Autodesk Inventor part; units mm, degrees
ref_plane "YZ Plane" through (0, 0, 0) normal (1, 0, 0) x (0, 1, 0)
ref_plane "XZ Plane" through (0, 0, 0) normal (0, 1, 0) x (-1, 0, 0)
ref_plane "XY Plane" through (0, 0, 0) normal (0, 0, 1) x (1, 0, 0)
sketch "草圖1" plane through (0, 0, 0) normal (0, 1, 0) x (-1, 0, 0)
  line L0 (0, 0) -> (20, 0)
  line L1 (20, 0) -> (20, 16)
  line L2 (20, 16) -> (0, 16)
  line L3 (0, 16) -> (0, 0)
  dimension "d0" = 20
  dimension "d1" = 16
extrude "擠出1" add sketch "草圖1" along normal blind 11.5
sketch "草圖2" plane through (-20, 0, 16) normal (0, 0, 1) x (1, 0, 0)
  line L0 (0, 0) -> (20, 0)
  line L1 (20, 0) -> (20, 11.5)
  point P0 (16.5, 4.8)
  dimension "d4" = 3.5
  dimension "d5" = 4.8
hole "孔1" at (-3.5, 4.8, 16) direction (0, 0, -1) diameter 2.459 depth 3.5 tip angle 118
sketch "草圖3" plane through (-20, 0, 16) normal (0, 0, 1) x (1, 0, 0)
  line L0 (0, 0) -> (20, 0)
  line L1 (20, 0) -> (20, 11.5)
  point P0 (18, 2)
  dimension "d13" = 2
  dimension "d14" = 2
hole "孔2" at (-2, 2, 16) direction (0, 0, -1) diameter 1.5 depth 4.5 tip angle 118
chamfer "倒角1" distance 0.5 angle 45 12 edges at (-10, 0, 16) (0, 5.75, 16) (0, 0, 8) (-20, 0, 8) (-20, 5.75, 16) (0, 5.75, 0) (-10, 0, 0) (0, 11.5, 8) (-10, 11.5, 16) (-20, 11.5, 8) (-20, 5.75, 0) (-10, 11.5, 0)
sketch "草圖4" plane through (-19.5, 0.5, 16) normal (0, 0, 1) x (1, 0, 0)
  circle A0 centre (8, 3.5) radius 3
  line L0 (0, -0.5) -> (19, -0.5)
  line L1 (-0.5, 4.5) -> (8, 4.5)
  line L2 (8, 4.5) -> (8, 2.5)
  line L3 (8, 2.5) -> (-0.5, 2.5)
  line L4 (-0.5, 2.5) -> (-0.5, 4.5)
  point P0 (19.5, -0.5)
  dimension "d25" = 6
  dimension "d27" = 11.5
  dimension "d28" = 4
  dimension "d29" = 2
  dimension "d30" = 8.5
extrude "擠出2" cut sketch "草圖4" against normal through all
sketch "草圖5" plane through (0, 0, 0) normal (0, -1, 0) x (1, 0, 0)
  point P0 (0, 0)
  point P1 (-17.5, 8)
  dimension "d35" = 17.5
hole "孔3" at (-17.5, 0, 8) direction (0, 1, 0) diameter 2.459 end through all
sketch "草圖6" plane through (0, 0, 0) normal (0, -1, 0) x (1, 0, 0)
  point P0 (0, 0)
  point P1 (-4.5, 8)
  dimension "d43" = 4.5
hole "孔4" at (-4.5, 0, 8) direction (0, 1, 0) diameter 4.917 end through all
properties part number "e3d_v6_heat_block"
Build history of the part. All positions in model axes, mm. A direction names the side the tool comes from. Coordinates: 2 decimals unless noted, no trailing zeros. Order: outer loops, then holes, each group sorted by start corner. A loop starts at its lowest first (then second) coordinate and runs counter-clockwise, first axis right, second up. Notation, with made-up numbers: (-34.75, 5.5) - (19.25, 5.5) arc R32 cw to (19.25, 39.5) - close; hole circle Ø1 at (44, 34). An arc over 180 degrees is marked (long way). Put each result on its own line as item: value.
1. Pull direction Z, two halves, no side cores. Call faces 1 (the face through (-10, 7, 16)), 2 (the face through (-10, 7, 0)), 3 (the face through (-18.72, 1.52, 8.16)): pulls with the +Z half, pulls with the -Z half, needs draft (parallel to the pull), parting line crosses it, or undercut.
Answer sheet:
face 1: pulls with the +Z half
face 2: pulls with the -Z half
face 3: undercut
2. Saw through at C-C (y = 9.25). Write the cut outline in (x, z), and give its area (3 significant figures).
Answer sheet:
outline: (-20, 0.5) - (-19.5, 0) - (-0.5, 0) - (0, 0.5) - (0, 15.5) - (-0.5, 16) - (-19.5, 16) - (-20, 15.5) - close; hole circle Ø2.46 at (-17.5, 8); hole circle Ø4.92 at (-4.5, 8)
area: 296 mm^2
3. Saw through at B-B (z = 12). Write the cut outline in (x, y), and give its area (3 significant figures).
Answer sheet:
outline: (-20, 0.5) - (-19.5, 0) - (-0.5, 0) - (0, 0.5) - (0, 11) - (-0.5, 11.5) - (-19.5, 11.5) - (-20, 11) - (-20, 5) - (-14.33, 5) arc R3 cw (long way) to (-14.33, 3) - (-20, 3) - close; hole circle Ø0.79 at (-3.5, 4.8); hole circle Ø1.5 at (-2, 2)
area: 188 mm^2
4. Tool access for faces 4 (the face through (-3.55, 6.03, 14.23)), 5 (the face through (-16, 3, 8)), 6 (the face through (-20, 8, 8)): list every direction of +Z, -Z, +X, -X, +Y, -Y with a clear straight run to the whole face (end or side of a thin tool).
Answer sheet:
face 4: +Z
face 5: +Z, -Z, -X
face 6: +Z, -Z, -X, +Y, -Y
5. Probe line 1 along X through (y, z) = (9.25, 8); line 2 along Y through (x, z) = (-18.5, 6.5); line 3 along Z through (x, y) = (-17.5, 0.95). List the from-to ranges inside material, lowest first. Write a range as [from, to].
Answer sheet:
line 1: x = [-20, -18.73], [-16.27, -6.96], [-2.04, 0]
line 2: y = [0, 3], [5, 11.5]
line 3: z = [0, 6.77], [9.23, 16]
6. Saw through at D-D (z = 8.75). Write the cut outline in (x, y), and give its area (3 significant figures).
Answer sheet:
outline: (-20, 0.5) - (-19.5, 0) - (-18.47, 0) - (-18.47, 3) - (-20, 3) - close; (-20, 5) - (-18.47, 5) - (-18.47, 11.5) - (-19.5, 11.5) - (-20, 11) - close; (-16.53, 0) - (-6.84, 0) - (-6.84, 11.5) - (-16.53, 11.5) - (-16.53, 5) - (-14.33, 5) arc R3 cw (long way) to (-14.33, 3) - (-16.53, 3) - close; (-2.16, 0) - (-0.5, 0) - (0, 0.5) - (0, 11) - (-0.5, 11.5) - (-2.16, 11.5) - close
area: 118 mm^2
7. Saw through at A-A (x = -11.5). Write the cut outline in (y, z).
Answer sheet:
outline: (0, 0.5) - (0.5, 0) - (1, 0) - (1, 16) - (0.5, 16) - (0, 15.5) - close; (7, 0) - (11, 0) - (11.5, 0.5) - (11.5, 15.5) - (11, 16) - (7, 16) - close
